from build123d import *

# Parameters (mm, degrees)
DODANIE_WYCI_GNI_CIE1_START = -40
DODANIE_WYCI_GNI_CIE1_DEPTH = 40
SZKIC4_R                    = 96
WYTNIJ_WYCI_GNI_CIE1_DEPTH  = 40


with BuildPart() as part:
    # Szkic1 → Obrót1 (revolve)
    with BuildSketch(Plane.XY):
        Polygon((-52.739893705, 77.020736352), (-92.739893705, 77.020736352), (-92.739893705, 88.020736352), (-83.110941126, 88.020736352), (-83.110941126, 96.020736352), (-92.739893705, 96.020736352), (-92.739893705, 107.020736352), (-52.739893705, 107.020736352), (-52.739893705, 96.020736352), (-62.368846284, 96.020736352), (-62.368846284, 88.020736352), (-52.739893705, 88.020736352), align=None)
    revolve(axis=Axis((0, 0, 0), (-1, 0, 0)))

    # Szkic2 → Dodanie-wyciągnięcie1 (add)
    with BuildSketch(Plane.ZY.offset(92.739893705).offset(DODANIE_WYCI_GNI_CIE1_START)):
        with BuildLine():
            ThreePointArc((-107.020736352, 0), (0, -107.020736352), (107.020736352, 0))
            Line((107.020736352, 0), (107.020736352, -232.057883899))
            Line((107.020736352, -232.057883899), (-107.020736352, -232.057883899))
            Line((-107.020736352, -232.057883899), (-107.020736352, 0))
        make_face()
    extrude(amount=DODANIE_WYCI_GNI_CIE1_DEPTH)

    # Szkic4 → Wytnij-wyciągnięcie1 (cut)
    with BuildSketch(Plane.ZY.offset(92.739893705)):
        with Locations(Location((0, 0, 0), (0, 0, 270))):
            Circle(SZKIC4_R)
    extrude(amount=-WYTNIJ_WYCI_GNI_CIE1_DEPTH, mode=Mode.SUBTRACT)


solid = part.part
The model under review builds one solid part; all positions refer to its coordinate system, in mm. Round coordinates to 2 decimals unless told otherwise and drop trailing zeros. Write each loop counter-clockwise with the first axis right and the second up, starting at its lowest first coordinate (ties: lowest second). Pieces come first, ordered by that corner, then holes. Notation, with made-up numbers: (30.25, 25) -> (52.25, 25) arc R23 cw to (52.25, 47) -> close; hole circle Ø6 at (67.25, 29.25). An arc over 180 degrees is marked (long way). Answer as a JSON object with one key per item and string values.
1. The part is to be moulded in two halves that separate along Z. For faces 1 (the face through (-72, -114, 107.021)), 2 (the face through (-52.74, -140, -1)), 3 (the face through (-87.993, 51.62, -80.965)), say which applies: pulls with the +Z half, pulls with the -Z half, needs draft (parallel to the pull), parting line crosses it, or undercut.
Results found:
{"face 1": "pulls with the +Z half", "face 2": "needs draft", "face 3": "undercut"}
2. We need section B-B on x = -86.5. State the section outline as (y, z) points, and give its area (3 significant figures).
Results found:
{"outline": "(-232.06, -107.02) -> (0, -107.02) arc R107.02 ccw to (0, 107.02) -> (-232.06, 107.02) -> close; hole circle Ø192.04 at (0, 0)", "area": "38,700 mm^2"}
3. Clearance check with flat-ended pins moving along their axes: pin 1 (8 mm diameter, centred on x = -64, y = 37.5, fed in from -Z); pin 2 (3 mm diameter, centred on x = -68.5, y = 11.5, fed in from -Z); pin 3 (2 mm diameter, centred on x = -67, z = -27, fed in from +Y). State where each tip first meets the part, or that it passes through.
Results found:
{"pin 1": "stops at z = -101.64", "pin 2": "stops at z = -106.55", "pin 3": "stops at y = 103.81"}
4. To check wall thickness, follow line 1 along Z through (x, y) = (-55, -3); line 2 along Y through (x, z) = (-59.75, 0); line 3 along Y through (x, z) = (-63.5, 53). State the ranges of each line that lie inside material, in increasing order.
Results found:
{"line 1": "z = -107.02 to -95.97, 95.97 to 107.02", "line 2": "y = -232.06 to -96.02, 96.02 to 107.02", "line 3": "y = -232.06 to -80.04, 80.04 to 92.98"}
